from build123d import *

# Parameters (mm, degrees)
ESQUISSE1_W             = 15
ESQUISSE1_H             = 40
BOSS_EXTRU_1_DEPTH      = 5
ESQUISSE2_W             = 6.8
ESQUISSE2_H             = 6.2
ENL_V_MAT_EXTRU_1_DEPTH = 4.2
ESQUISSE3_W             = 0.8
ESQUISSE3_H             = 1.2
ENL_V_MAT_EXTRU_2_DEPTH = 22.769014677
CHANFREIN1_SIZE         = 2


with BuildPart() as part:
    # Esquisse1 → Boss.-Extru.1 (new body)
    with BuildSketch(Plane.XY):
        Rectangle(ESQUISSE1_W, ESQUISSE1_H)
    extrude(amount=BOSS_EXTRU_1_DEPTH)

    # Esquisse2 → Enlèv. mat.-Extru.1 (cut)
    with BuildSketch(Plane.XY.offset(5)):
        with Locations((0, -2.5)):
            Rectangle(ESQUISSE2_W, ESQUISSE2_H)
        with Locations((0, 12.5)):
            Rectangle(ESQUISSE2_W, ESQUISSE2_H)
        with Locations((0, -12.5)):
            Rectangle(ESQUISSE2_W, ESQUISSE2_H)
    extrude(amount=-ENL_V_MAT_EXTRU_1_DEPTH, mode=Mode.SUBTRACT)

    # Esquisse3 → Enlèv. mat.-Extru.2 (cut, through all)
    with BuildSketch(Plane.XY.offset(0.8)):
        with Locations((-3, 0)):
            Rectangle(ESQUISSE3_W, ESQUISSE3_H)
        with Locations((-3, 10)):
            Rectangle(ESQUISSE3_W, ESQUISSE3_H)
        with Locations((-3, 15)):
            Rectangle(ESQUISSE3_W, ESQUISSE3_H)
        with Locations((3, 15)):
            Rectangle(ESQUISSE3_W, ESQUISSE3_H)
        with Locations((3, 10)):
            Rectangle(ESQUISSE3_W, ESQUISSE3_H)
        with Locations((3, 0)):
            Rectangle(ESQUISSE3_W, ESQUISSE3_H)
        with Locations((3, -5)):
            Rectangle(ESQUISSE3_W, ESQUISSE3_H)
        with Locations((3, -15)):
            Rectangle(ESQUISSE3_W, ESQUISSE3_H)
        with Locations((3, -10)):
            Rectangle(ESQUISSE3_W, ESQUISSE3_H)
        with Locations((-3, -10)):
            Rectangle(ESQUISSE3_W, ESQUISSE3_H)
        with Locations((-3, -15)):
            Rectangle(ESQUISSE3_W, ESQUISSE3_H)
        with Locations((-3, -5)):
            Rectangle(ESQUISSE3_W, ESQUISSE3_H)
    extrude(amount=-ENL_V_MAT_EXTRU_2_DEPTH, mode=Mode.SUBTRACT)

    # Chanfrein1
    chanfrein1_edges = [part.edges().sort_by_distance(p)[0] for p in [
        (0, -20, 0),
        (-7.5, 0, 0),
        (0, 20, 0),
        (7.5, 0, 0),
    ]]
    chamfer(chanfrein1_edges, length=CHANFREIN1_SIZE)


solid = part.part
Model file for the job. Use its own axes, mm. A direction names the side the tool comes from. Give positions to 0.01 mm unless a question says otherwise; leave off trailing zeros. Loops run counter-clockwise (first coordinate to the right, second up) from the corner with the lowest first, then second, coordinate; pieces in that order, holes last.
Item 1: Slice it at A-A (z = 3.8). Write the cut outline in (x, y).
Check values:
outline: (-7.5, -20) - (7.5, -20) - (7.5, 20) - (-7.5, 20) - close; hole (-3.4, -15.6) - (3.4, -15.6) - (3.4, -9.4) - (-3.4, -9.4) - close; hole (-3.4, -5.6) - (3.4, -5.6) - (3.4, 0.6) - (-3.4, 0.6) - close; hole (-3.4, 9.4) - (3.4, 9.4) - (3.4, 15.6) - (-3.4, 15.6) - close
Item 2: Slice it at C-C (y = 11). Write the cut outline in (x, z), plus the area to 3 significant figures.
Check values:
outline: (-7.5, 2) - (-5.5, 0) - (5.5, 0) - (7.5, 2) - (7.5, 5) - (3.4, 5) - (3.4, 0.8) - (-3.4, 0.8) - (-3.4, 5) - (-7.5, 5) - close
area: 42.4 mm2
Item 3: Which spindle directions (+Z, -Z, +X, -X, +Y, -Y) get a long thin tool onto all of the face, cutting with end or side? Do faces 1 (the face through (-3.4, -13, 3)), 2 (the face through (0, -19, 1)). Say none if no direction does.
Check values:
face 1: +Z
face 2: -Z, +X, -X, -Y
Item 4: Mould opens along X. For faces 3 (the face through (0, 0, 0)), 4 (the face through (0, -15.6, 3)), 5 (the face through (6.5, -0.3, 1)) say: +X half, -X half, draft (parallel to the pull), parting line (faces both ways), or undercut.
Check values:
face 3: draft
face 4: undercut
face 5: +X half
Item 5: Drop flat-ended pins along their axis: P1, Ø0.6, axis at y = 10, z = 0.5, coming from the +X side; P2, Ø0.9, axis at y = 0, z = 0.5, coming from the +X side. Give the stop position or say it passes through.
Check values:
P1: stops at x = 6.3
P2: stops at x = 6.45
Item 6: Slice it at D-D (z = 1.3). Write the cut outline in (x, y), plus the area to 3 significant figures.
Check values:
outline: (-6.8, -19.3) - (6.8, -19.3) - (6.8, 19.3) - (-6.8, 19.3) - close; hole (-3.4, -15.6) - (3.4, -15.6) - (3.4, -9.4) - (-3.4, -9.4) - close; hole (-3.4, -5.6) - (3.4, -5.6) - (3.4, 0.6) - (-3.4, 0.6) - close; hole (-3.4, 9.4) - (3.4, 9.4) - (3.4, 15.6) - (-3.4, 15.6) - close
area: 398 mm2
Item 7: Slice it at B-B (y = -15). Write the cut outline in (x, z).
Check values:
outline: (-7.5, 2) - (-5.5, 0) - (-3.4, 0) - (-3.4, 5) - (-7.5, 5) - close; (-2.6, 0) - (2.6, 0) - (2.6, 0.8) - (-2.6, 0.8) - close; (3.4, 0) - (5.5, 0) - (7.5, 2) - (7.5, 5) - (3.4, 5) - close
Item 8: Drill centre lines: line 1 along Y through (x, z) = (-1.25, 2.6); line 2 along X through (y, z) = (0.5, 3.65); line 3 along X through (y, z) = (-10.5, 0.6). Where is each one in solid material? Low to high.
Check values:
line 1: y = -20 to -15.6, -9.4 to -5.6, 0.6 to 9.4, 15.6 to 20
line 2: x = -7.5 to -3.4, 3.4 to 7.5
line 3: x = -6.1 to -3.4, -2.6 to 2.6, 3.4 to 6.1
